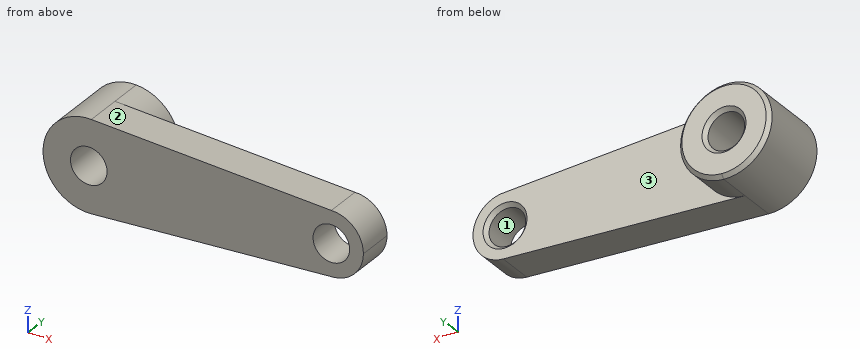
```python
from build123d import *

# Parameters (mm, degrees)
F0_R     = 10
F1_DEPTH = 20
F2_DEPTH = 20
F3_SIZE  = 2


with BuildPart() as f1:
    # F0 (on Front) → F1 (new body)
    with BuildSketch(Plane.XZ):
        with BuildLine():
            ThreePointArc((1.415094, -24.959918), (18.171095, -17.17007), (25, 0))
            ThreePointArc((25, 0), (18.172929, 17.168129), (1.420428, 24.959615))
            ThreePointArc((1.420428, 24.959615), (-25, 0.002671), (1.415094, -24.959918))
        make_face()
        Circle(F0_R, mode=Mode.SUBTRACT)
        with BuildLine():
            ThreePointArc((1.420428, 24.959615), (18.172929, 17.168129), (25, 0))
            ThreePointArc((25, 0), (18.171095, -17.17007), (1.415094, -24.959918))
            Line((1.415094, -24.959918), (133.490566, -17.471943))
            ThreePointArc((133.490566, -17.471943), (115.007016, -0.495482), (132.5, 17.5))
            Line((132.5, 17.5), (1.420428, 24.959615))
        make_face()
        with BuildLine():
            ThreePointArc((150, 0), (144.874369, 12.374369), (132.5, 17.5))
            ThreePointArc((132.5, 17.5), (115.007016, -0.495482), (133.490566, -17.471943))
            ThreePointArc((133.490566, -17.471943), (145.219766, -12.019049), (150, 0))
        make_face()
        with Locations((132.5, 0)):
            Circle(F0_R, mode=Mode.SUBTRACT)
    extrude(amount=F1_DEPTH)

    # F0 (on Front) → F2 (join)
    with BuildSketch(Plane.XZ):
        with BuildLine():
            ThreePointArc((1.415094, -24.959918), (18.171095, -17.17007), (25, 0))
            ThreePointArc((25, 0), (18.172929, 17.168129), (1.420428, 24.959615))
            ThreePointArc((1.420428, 24.959615), (-25, 0.002671), (1.415094, -24.959918))
        make_face()
        Circle(F0_R, mode=Mode.SUBTRACT)
    extrude(amount=-F2_DEPTH)

    # F3
    f3_edges = [f1.edges().sort_by_distance(p)[0] for p in [
        (-10, 20, 0),
        (-1.415094, 20, 24.959918),
        (122.5, 0, 0),
    ]]
    chamfer(f3_edges, length=F3_SIZE)


solid = f1.part
```
Design review of the part built by this model. Coordinates are the model's own, in mm. Face numbers are marked on the shaded views. Coordinates: 2 decimals unless noted, no trailing zeros. Write each loop counter-clockwise with the first axis right and the second up, starting at its lowest first coordinate (ties: lowest second). Pieces come first, ordered by that corner, then holes.
1) To check wall thickness, follow L1, parallel to X at y = 13.5, z = 0.5 (1 decimal); L2, parallel to Y at x = 47, z = 18. State the ranges of each line that lie inside material, in increasing order.
2) Add section C-C (x = 102). Write out the cut boundary in (y, z), plus the area to 3 significant figures.
3) Mouldability with a two-part tool opening along Z and no side actions: class the marked faces 1, 2 and 3 as +Z half, -Z half, draft (parallel to the pull), parting line (faces both ways), or undercut.
4) Add section D-D (x = 53). Write out the cut boundary in (y, z).
5) Insertion check: pin 1 (3 mm diameter, centred on y = -16, z = 6, fed in from +X); pin 2 (3 mm diameter, centred on x = 71, z = 13.5, fed in from +Y); pin 3 (18 mm diameter, centred on x = 0, z = 0, fed in from -Y); pin 4 (8 mm diameter, centred on x = 11.5, y = 3, fed in from +Z). Each pin has a flat end and moves straight along its axis. Give the tip position at first contact, or say it passes through.
6) Add section B-B (z = -3.5). State how many separate pieces and enclosed holes the cut face has, plus the area to 3 significant figures.
7) Add section A-A (y = 2.5). Write out the cut boundary in (x, z).
Check result:
1. L1: x = -25 to -10, 10 to 25
1. L2: y = -20 to 0
2. outline: (-20, -19.26) - (0, -19.26) - (0, 19.24) - (-20, 19.24) - close
2. area: 770 mm2
3. face 1: undercut
3. face 2: +Z half
3. face 3: draft
4. outline: (-20, -22.04) - (0, -22.04) - (0, 22.02) - (-20, 22.02) - close
5. pin 1: stops at x = 149.41
5. pin 2: stops at y = 0
5. pin 3: passes through
5. pin 4: stops at z = 24.54
6. separate pieces: 3
6. enclosed holes: 0
6. area: 3,340 mm2
7. outline: circle Ø50 at (0, 0); hole circle Ø20 at (0, 0)
